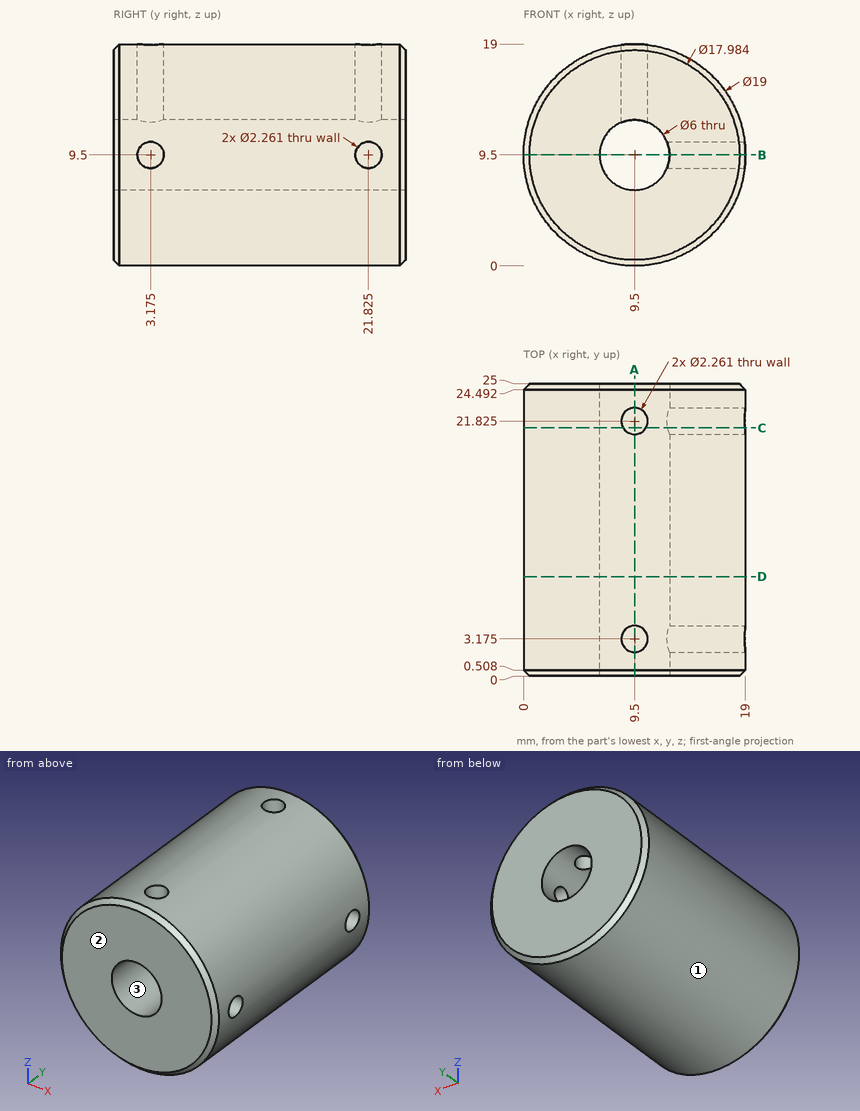
For this review, use the dimensioned drawing (mm, ordinates from the lowest corner) and the shaded views. Give positions to 0.01 mm unless a question says otherwise; leave off trailing zeros. Loops run counter-clockwise (first coordinate to the right, second up) from the corner with the lowest first, then second, coordinate; pieces in that order, holes last. Notation, with made-up numbers: (79.5, 81) - (115.5, 81) arc R15 cw to (115.5, 87) - close; hole circle Ø9 at (-38.5, 10.25). An arc over 180 degrees is marked (long way). Write each question's results on one line, items separated by ' | '.
(1) For pin 1 Ø2 at (x, y) = (9.5, 21.825) entering from +Z; pin 2 Ø10 at (x, y) = (15, 9) entering from -Z; pin 3 Ø1.4 at (y, z) = (3.175, 9.5) entering from +X, all flat-tipped, find the tip position at first contact; note any pin that passes through.
Conclusion:
pin 1: z = 6.67 | pin 2: z = 0.01 | pin 3: x = 6.58
(2) Take a section at D-D (y = 8.5). Give the boundary of the cut face in (x, z).
Conclusion:
outline: circle Ø19 at (9.5, 9.5); hole circle Ø6 at (9.5, 9.5)
(3) Draft analysis for pull direction Z (two halves, no side actions). For the marked faces 1, 2 and 3, state which applies: +Z half, -Z half, draft (parallel to the pull), parting line (faces both ways), or undercut.
Conclusion:
face 1: parting line | face 2: draft | face 3: undercut
(4) Take a section at A-A (x = 9.5). Give the boundary of the cut face in (y, z) (1 decimal), then the cut area to 3 significant figures.
Conclusion:
outline: (0, 0.5) - (0.5, 0) - (24.5, 0) - (25, 0.5) - (25, 6.5) - (0, 6.5) - close; (0, 12.5) - (2, 12.5) - (2, 19) - (0.5, 19) - (0, 18.5) - close; (4.3, 12.5) - (20.7, 12.5) - (20.7, 19) - (4.3, 19) - close; (23, 12.5) - (25, 12.5) - (25, 18.5) - (24.5, 19) - (23, 19) - close | area: 295 mm^2
(5) Take a section at C-C (y = 21.25). Give the boundary of the cut face in (x, z).
Conclusion:
outline: (8.53, 12.34) - (8.53, 18.95) arc R9.5 ccw (long way) to (18.95, 8.53) - (12.34, 8.53) arc R3 cw (long way) to start; (10.47, 12.34) arc R3 cw to (12.34, 10.47) - (18.95, 10.47) arc R9.5 ccw to (10.47, 18.95) - close
(6) For line 1 along Y through (x, z) = (17, 9.5) (1 decimal); line 2 along Y through (x, z) = (9.75, 17.75); line 3 along X through (y, z) = (19, 7.25) (1 decimal), list the stretches that pass through material, from the lowest coordinate up.
Conclusion:
line 1: 0 to 2, 4.3 to 20.7, 23 to 25 | line 2: 0 to 2.07, 4.28 to 20.72, 22.93 to 25 | line 3: 0.3 to 7.5, 11.5 to 18.7
(7) Take a section at B-B (z = 9.5). Give the boundary of the cut face in (x, y) (1 decimal).
Conclusion:
outline: (0, 0.5) - (0.5, 0) - (6.5, 0) - (6.5, 25) - (0.5, 25) - (0, 24.5) - close; (12.5, 0) - (18.5, 0) - (19, 0.5) - (19, 2) - (12.5, 2) - close; (12.5, 4.3) - (19, 4.3) - (19, 20.7) - (12.5, 20.7) - close; (12.5, 23) - (19, 23) - (19, 24.5) - (18.5, 25) - (12.5, 25) - close
